Could you check a few things on this model? Use its own coordinates, in mm. Give positions to 0.01 mm unless a question says otherwise; leave off trailing zeros. Loops run counter-clockwise (first coordinate to the right, second up) from the corner with the lowest first, then second, coordinate; pieces in that order, holes last. Notation, with made-up numbers: (82, 67) - (99, 67) arc R25 cw to (99, 80) - close; hole circle Ø8 at (-8.5, 86.5). An arc over 180 degrees is marked (long way). One line per item, written item: value. Start each with the question number.
Q1. I'm going to push flat-ended pins straight in: P1, Ø2, axis at x = -3.5, z = 7.5, coming from the -Y side; P2, Ø5, axis at x = 5.5, z = 5, coming from the -Y side. Where does each tip first touch, or does it pass through?
Q2. If I drill on line 1 (Y direction, x = 0, z = 3.25); line 2 (X direction, y = -180, z = 6); line 3 (Y direction, x = -2.5, z = 9.5), over which ranges is the centre line in solid material (lowest first)? Write a range as from..to.
Q3. If we mould it in two halves opening along Y, with no side actions, what happens to faces 1 (the face through (-0.651, -184.957, 4.93)), 2 (the face through (0, -190, 5)), 3 (the face through (0, 10, 5)), 4 (the face through (-10, -89, 5))? For each: released by +Y, released by -Y, zero draft, split by the parting line, or undercut.
Q4. I want a section at B-B (z = 5.25). Please give me the cut outline in (x, y).
Q5. I want a section at A-A (x = 0). Please give me the cut outline in (y, z), then the cut area to 3 significant figures.
Autodesk Inventor part; units mm, degrees
ref_plane "YZ Plane" through (0, 0, 0) normal (1, 0, 0) x (0, 1, 0)
ref_plane "XZ Plane" through (0, 0, 0) normal (0, 1, 0) x (-1, 0, 0)
ref_plane "XY Plane" through (0, 0, 0) normal (0, 0, 1) x (1, 0, 0)
sketch "スケッチ1" plane through (0, 0, 0) normal (0, 0, 1) x (1, 0, 0)
  circle A0 centre (0, 0) radius 5
  circle A1 centre (0, 0) radius 10
  line L0 (-5, 0) -> (5, 0)
  line L1 (5, 0) -> (5, -190)
  line L2 (5, -190) -> (-5, -190)
  line L3 (-5, -190) -> (-5, 0)
  line L4 (-10, 0) -> (-10, -190)
  line L5 (-10, -190) -> (5, -190)
  line L6 (10, 0) -> (10, -190)
  line L7 (10, -190) -> (5, -190)
  circle A2 centre (0, -180) radius 5
  circle A3 centre (0, -180) radius 10
  point P0 (5, -8.6603)
  point P1 (-5, -8.6603)
  point P2 (-5, -171.3397)
  point P3 (5, -171.3397)
  point P4 (-10, -180)
  point P5 (10, -180)
  dimension "d0" = 10
  dimension "d1" = 20
  dimension "d3" = 10
  dimension "d15" = 20
  dimension "d16" = 10
  dimension "d17" = 20
  dimension "d18" = 10
  dimension "d19" = 10
  dimension "d22" = 180
extrude "押し出し1" add sketch "スケッチ1" along normal blind 10 contours L1 A1 L3 A0 | A0 L3 A1 L1 | L1 A3 L3 A1 | A1 L6 A3 L1 | L3 A3 L4 A1 | A3 L1 | L1 A2 L3 A3 | L3 A3 | L1 A3 L3 A2
properties part number "legparts_03(six)"
Worked answers:
1. P1: stops at y = -189.68
1. P2: stops at y = -189.54
2. line 1: y = -190..-185, -175..-5, 5..10
2. line 2: x = -10..-5, 5..10
2. line 3: y = -189.68..-184.33, -175.67..-4.33, 4.33..9.68
3. face 1: undercut
3. face 2: released by -Y
3. face 3: released by +Y
3. face 4: zero draft
4. outline: (-10, -180) arc R10 ccw to (10, -180) - (10, 0) arc R10 ccw to (-10, 0) - close; hole circle Ø10 at (0, -180); hole circle Ø10 at (0, 0)
5. outline: (-190, 0) - (-185, 0) - (-185, 10) - (-190, 10) - close; (-175, 0) - (-5, 0) - (-5, 10) - (-175, 10) - close; (5, 0) - (10, 0) - (10, 10) - (5, 10) - close
5. area: 1,800 mm²
